Model file for the job. Use its own axes, mm. Face numbers are marked on the shaded views. A direction names the side the tool comes from. Give positions to 0.01 mm unless a question says otherwise; leave off trailing zeros. Write each loop counter-clockwise with the first axis right and the second up, starting at its lowest first coordinate (ties: lowest second). Pieces come first, ordered by that corner, then holes. Notation, with made-up numbers: (-8.5, 12.25) - (4.5, 12.25) arc R25 ccw to (4.5, 34.25) - close; hole circle Ø3 at (-17.5, 77.25). An arc over 180 degrees is marked (long way). Use a Markdown table: item, result. Add a question column.
```python
from build123d import *

# Parameters (mm, degrees)
F0_W      = 50.8
F0_H      = 57.15
F1_DEPTH  = 31.75
F2_W      = 50.8
F2_H      = 50.8
F3_DEPTH  = 6.35
F4_DEPTH  = 12.7
F6_DEPTH  = 25.4
F8_DEPTH  = 12.7
F9_DEPTH  = 25.4
F10_R     = 6.35
F11_DEPTH = 50.8
F12_R     = 3.175
F13_DEPTH = 25.4


with BuildPart() as f1:
    # F0 (on Front) → F1 (new body)
    with BuildSketch(Plane.XZ):
        with Locations((6.0355709866, -8.0190159138)):
            Rectangle(F0_W, F0_H)
    extrude(amount=F1_DEPTH)

    # F2 (on face) → F3 (join)
    with BuildSketch(Plane.XZ.offset(31.75)):
        with Locations((6.0355709866, -4.8440159138)):
            Rectangle(F2_W, F2_H)
    extrude(amount=F3_DEPTH)

    # F4 (cut): a face of the model
    f4_faces = [f1.faces().sort_by_distance(p)[0] for p in [
        (6.0355709866, -38.1, -4.8440159138),
    ]]
    extrude(f4_faces, amount=-F4_DEPTH, mode=Mode.SUBTRACT)

    # F5 (on face) → F6 (cut)
    with BuildSketch(Plane.XZ.offset(25.4)):
        with BuildLine():
            Line((-6.6644290134, -17.5440159138), (-6.6644290134, 20.5559840862))
            Line((-6.6644290134, 20.5559840862), (-19.3644290134, 20.5559840862))
            Line((-19.3644290134, 20.5559840862), (-19.3644290134, -30.2440159138))
            ThreePointArc((-19.3644290134, -30.2440159138), (-10.3841728924, -26.5242720349), (-6.6644290134, -17.5440159138))
        make_face()
        with BuildLine():
            Line((31.4355709866, 20.5559840862), (18.7355709866, 20.5559840862))
            Line((18.7355709866, 20.5559840862), (18.7355709866, -17.5440159138))
            ThreePointArc((18.7355709866, -17.5440159138), (22.4553148655, -26.5242720349), (31.4355709866, -30.2440159138))
            Line((31.4355709866, -30.2440159138), (31.4355709866, 20.5559840862))
        make_face()
    extrude(amount=-F6_DEPTH, mode=Mode.SUBTRACT)

    # F7 (on face) → F8 (cut)
    with BuildSketch(Plane.XZ.offset(25.4)):
        with BuildLine():
            ThreePointArc((6.0355709866, -4.8440159138), (-2.9446851345, -1.1242720349), (-6.6644290134, 7.8559840862))
            Line((-6.6644290134, 7.8559840862), (-6.6644290134, -17.5440159138))
            ThreePointArc((-6.6644290134, -17.5440159138), (-10.3841728924, -26.5242720349), (-19.3644290134, -30.2440159138))
            Line((-19.3644290134, -30.2440159138), (31.4355709866, -30.2440159138))
            ThreePointArc((31.4355709866, -30.2440159138), (22.4553148655, -26.5242720349), (18.7355709866, -17.5440159138))
            Line((18.7355709866, -17.5440159138), (18.7355709866, 7.8559840862))
            ThreePointArc((18.7355709866, 7.8559840862), (15.0158271076, -1.1242720349), (6.0355709866, -4.8440159138))
        make_face()
        with BuildLine():
            Line((18.7355709866, 20.5559840862), (6.0355709866, 20.5559840862))
            ThreePointArc((6.0355709866, 20.5559840862), (15.0158271076, 16.8362402072), (18.7355709866, 7.8559840862))
            Line((18.7355709866, 7.8559840862), (18.7355709866, 20.5559840862))
        make_face()
        with BuildLine():
            ThreePointArc((-6.6644290134, 7.8559840862), (-2.9446851345, 16.8362402072), (6.0355709866, 20.5559840862))
            Line((6.0355709866, 20.5559840862), (-6.6644290134, 20.5559840862))
            Line((-6.6644290134, 20.5559840862), (-6.6644290134, 7.8559840862))
        make_face()
    extrude(amount=-F8_DEPTH, mode=Mode.SUBTRACT)

    # F9 (cut): faces of the model
    f9_faces = [f1.faces().sort_by_distance(p)[0] for p in [
        (15.898798162, -12.7, 17.7192112615),
        (-3.8276561888, -12.7, 17.7192112615),
    ]]
    extrude(f9_faces, amount=-F9_DEPTH, mode=Mode.SUBTRACT)

    # F10 (on face) → F11 (cut)
    with BuildSketch(Plane.XZ.offset(25.4)):
        with Locations((6.0355709866, 7.8559840862)):
            Circle(F10_R)
    extrude(amount=-F11_DEPTH, mode=Mode.SUBTRACT)

    # F12 (on face) → F13 (cut)
    with BuildSketch(Plane.XY.offset(-30.2440159138)):
        with Locations((-9.8394290134, -22.225)):
            Circle(F12_R)
        with BuildLine():
            ThreePointArc((-13.0144290134, -31.75), (-17.504557074, -29.8901280605), (-19.3644290134, -25.4))
            Line((-19.3644290134, -25.4), (-19.3644290134, -31.75))
            Line((-19.3644290134, -31.75), (-13.0144290134, -31.75))
        make_face()
        with Locations((21.9105709866, -22.225)):
            Circle(F12_R)
        with BuildLine():
            Line((31.4355709866, -31.75), (31.4355709866, -25.4))
            ThreePointArc((31.4355709866, -25.4), (29.5756990471, -29.8901280605), (25.0855709866, -31.75))
            Line((25.0855709866, -31.75), (31.4355709866, -31.75))
        make_face()
    extrude(amount=-F13_DEPTH, mode=Mode.SUBTRACT)


solid = f1.part
```
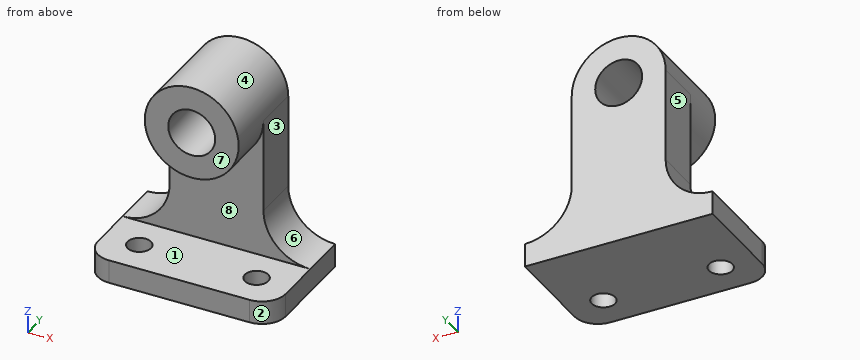
(1) Which spindle directions (+Z, -Z, +X, -X, +Y, -Y) get a long thin tool onto all of the face, cutting with end or side? Do the marked faces 1, 2, 3, 4 and 5. Say none if no direction does.
(2) Band-saw the part on C-C (y = -17.5). Write the cut outline in (x, z).
(3) Band-saw the part on B-B (z = 12). Write the cut outline in (x, y).
(4) Flat gauge pins, fed straight in: pin 1 (3 mm diameter, centred on y = -19.5, z = 3, fed in from +X); pin 2 (10 mm diameter, centred on y = -19, z = 5, fed in from -X); pin 3 (4 mm diameter, centred on x = 21.91, y = -22.22, fed in from -Z); pin 4 (9.5 mm diameter, centred on x = 12, y = -25, fed in from +Z). Where does each tip first touch, or does it go through?
(5) Probe probe 1 along Z at (x, y) = (11, -21.5); probe 2 along Z at (x, y) = (0.5, -24.5); probe 3 along Z at (x, y) = (8, -5.5). List the from-to ranges inside material, lowest first. Write a range as [from, to].
(6) Band-saw the part on D-D (y = -6). Write the cut outline in (x, z).
(7) Two-plate mould, pull along Z, no slides. Class the marked faces 6, 7 and 8: +Z half, -Z half, draft (parallel to the pull), parting line (faces both ways), or undercut.
(8) Band-saw the part on A-A (x = -11.5). Write the cut outline in (y, z).
Model answer:
| question | item | result |
|---|---|---|
| 1 | face 1 | +X, -X, -Y |
| 1 | face 2 | +Z, -Z, +X, -Y |
| 1 | face 3 | +Z, +X, +Y, -Y |
| 1 | face 4 | -Y |
| 1 | face 5 | +Z, -X, +Y, -Y |
| 2 | outline | (-19.36, -36.59) - (31.44, -36.59) - (31.44, -30.24) - (-19.36, -30.24) - close; circle Ø25.4 at (6.04, 7.86); hole circle Ø12.7 at (6.04, 7.86) |
| 3 | outline | (-5.97, -25.4) - (1.22, -25.4) - (1.22, 0) - (-5.97, 0) - close; (10.85, -25.4) - (18.04, -25.4) - (18.04, 0) - (10.85, 0) - close |
| 4 | pin 1 | stops at x = 18.28 |
| 4 | pin 2 | stops at x = -6.66 |
| 4 | pin 3 | passes through |
| 4 | pin 4 | stops at z = 20.5 |
| 5 | probe 1 | z = [-36.59, -30.24], [-3.83, 3.9], [11.82, 19.55] |
| 5 | probe 2 | z = [-36.59, -30.24], [-3.57, 4.74], [10.97, 19.29] |
| 5 | probe 3 | z = [-36.59, 1.82], [13.89, 20.4] |
| 6 | outline | (-19.36, -36.59) - (31.44, -36.59) - (31.44, -30.24) arc R12.7 cw to (18.74, -17.54) - (18.74, 7.86) arc R12.7 ccw to (-6.66, 7.86) - (-6.66, -17.54) arc R12.7 cw to (-19.36, -30.24) - close; hole circle Ø12.7 at (6.04, 7.86) |
| 7 | face 6 | +Z half |
| 7 | face 7 | draft |
| 7 | face 8 | undercut |
| 8 | outline | (-31.75, -36.59) - (-24.93, -36.59) - (-24.93, -30.24) - (-31.75, -30.24) - close; (-19.52, -36.59) - (0, -36.59) - (0, -27.52) - (-12.7, -27.52) - (-12.7, -30.24) - (-19.52, -30.24) - close |
